Verification items for the finished model (mm, model axes). Face numbers are marked on the shaded views. A direction names the side the tool comes from. Give positions to 0.01 mm unless a question says otherwise; leave off trailing zeros. Loops run counter-clockwise (first coordinate to the right, second up) from the corner with the lowest first, then second, coordinate; pieces in that order, holes last. Notation, with made-up numbers: M 14,0 L 51,0 A31 ccw 51,30 Z; hole C 52,-34.75 d9. An arc over 180 degrees is marked long. Use CSV: the item, a comma, the result in double quotes.
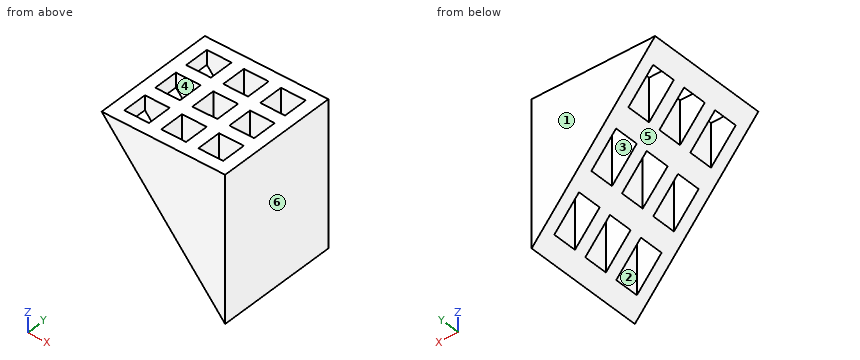
from build123d import *

# Parameters (mm, degrees)
F0_W     = 10
F0_H     = 10
F1_DEPTH = 577
F2_W     = 2
F2_H     = 2
F3_DEPTH = 577.001
F4_W     = 1.9998123646
F4_H     = 2
F4_W_2   = 2
F5_DEPTH = 577.001
F6_DEPTH = 500
F7_DEPTH = 65.276
F9_DEPTH = 10.001


with BuildPart() as f1:
    # F0 (on Top) → F1 (new body)
    with BuildSketch(Plane.XY):
        with Locations((-18.2401322573, 3.4046052024)):
            Rectangle(F0_W, F0_H)
    extrude(amount=F1_DEPTH)

    # F2 (on face) → F3 (cut, through all)
    with BuildSketch(Plane.XY.offset(577)):
        with Locations((-21.2401322573, 6.4046052024)):
            Rectangle(F2_W, F2_H)
        with Locations((-18.2401322573, 6.4046052024)):
            Rectangle(F2_W, F2_H)
        with Locations((-15.2401322573, 6.4046052024)):
            Rectangle(F2_W, F2_H)
        with Locations((-15.2401322573, 0.4046052024)):
            Rectangle(F2_W, F2_H)
        with Locations((-18.2401322573, 0.4046052024)):
            Rectangle(F2_W, F2_H)
        with Locations((-21.2401322573, 0.4046052024)):
            Rectangle(F2_W, F2_H)
    extrude(amount=-F3_DEPTH, mode=Mode.SUBTRACT)

    # F4 (on face) → F5 (cut, through all)
    with BuildSketch(Plane.XY.offset(577)):
        with Locations((-21.2402260751, 3.4046052024)):
            Rectangle(F4_W, F4_H)
        Polygon((-17.2403198928, 4.4376994483), (-19.2403198928, 4.4376994483), (-19.2403198928, 2.4046052024), (-17.2403198928, 2.4376994483), align=None)
        with Locations((-15.2403198928, 3.4074539542)):
            Rectangle(F4_W_2, F4_H)
    extrude(amount=-F5_DEPTH, mode=Mode.SUBTRACT)

    # F6 (cut): a face of the model
    f6_faces = [f1.faces().sort_by_distance(p)[0] for p in [
        (-13.3815536136, 3.4046052024, 577),
    ]]
    extrude(f6_faces, amount=-F6_DEPTH, mode=Mode.SUBTRACT)

    # F7 (cut): a face of the model
    f7_faces = [f1.faces().sort_by_distance(p)[0] for p in [
        (-13.3815536136, 3.4046052024, 77),
    ]]
    extrude(f7_faces, amount=-F7_DEPTH, mode=Mode.SUBTRACT)

    # F8 (on face) → F9 (cut, through all)
    with BuildSketch(Plane(origin=(0, 8.4046052024, 0), x_dir=(-1, 0, 0), z_dir=(0, 1, 0))):
        Polygon((23.2401322573, 0), (23.2401322573, 11.724), (13.2401322573, 0), align=None)
    extrude(amount=-F9_DEPTH, mode=Mode.SUBTRACT)


solid = f1.part
(1) Tool access check on the marked faces 1 and 2. Record the directions out of +Z, -Z, +X, -X, +Y, -Y that give a thin tool (end or side, any length) a straight path to the whole face; none if there is none.
Calculated:
face 1,"+Z, -Z, +X, -X, +Y"
face 2,"+Z, -Z"
(2) Depth check by flat-ended pin: pin 1 Ø5 at (y, z) = (3, 9.5) entering from -X; pin 2 Ø1.5 at (y, z) = (6, 9.5) entering from -X; pin 3 Ø6 at (y, z) = (2, 4.5) entering from -X. Enter the tip coordinate at first touch or a pass-through.
Calculated:
pin 1,"stops at x = -23.24"
pin 2,"stops at x = -21.73"
pin 3,"stops at x = -19.64"
(3) Scan lines: L1, parallel to X at y = 6.5, z = 8.5; L2, parallel to Y at x = -15, z = 2.5; L3, parallel to X at y = 2.75, z = 5.5. Record each from-to range of solid material in increasing order. Write a range as from..to.
Calculated:
L1,"x = -20.24..-19.24, -17.24..-16.24, -14.24..-13.24"
L2,"y = -1.6..-0.6, 1.4..2.41, 4.41..5.4, 7.4..8.4"
L3,"x = -17.24..-16.24, -14.24..-13.24"
(4) Section check A-A on y = 1. Record the cut outline in (x, z), plus the area to 3 significant figures.
Calculated:
outline,"M -23.24,11.72 L -22.24,10.55 L -22.24,11.72 Z; M -20.24,8.21 L -19.24,7.03 L -19.24,11.72 L -20.24,11.72 Z; M -17.24,4.69 L -16.24,3.52 L -16.24,11.72 L -17.24,11.72 Z; M -14.24,1.17 L -13.24,0 L -13.24,11.72 L -14.24,11.72 Z"
area,"23.4 mm²"
(5) Mould release check, pull along X, two halves, no side actions. Record for the marked faces 3, 4, 5 and 6: released by +X, released by -X, zero draft, split by the parting line, or undercut.
Calculated:
face 3,"undercut"
face 4,"undercut"
face 5,"released by -X"
face 6,"released by +X"
(6) Section check B-B on x = -14.75. Record the cut outline in (y, z), plus the area to 3 significant figures.
Calculated:
outline,"M -1.6,1.77 L -0.6,1.77 L -0.6,11.72 L -1.6,11.72 Z; M 1.4,1.77 L 2.41,1.77 L 2.41,11.72 L 1.4,11.72 Z; M 4.41,1.77 L 5.4,1.77 L 5.4,11.72 L 4.41,11.72 Z; M 7.4,1.77 L 8.4,1.77 L 8.4,11.72 L 7.4,11.72 Z"
area,"39.8 mm²"
(7) Section check C-C on z = 5.5. Record the cut outline in (x, y), plus the area to 3 significant figures.
Calculated:
outline,"M -17.93,-1.6 L -13.24,-1.6 L -13.24,8.4 L -17.93,8.4 L -17.93,7.4 L -17.24,7.4 L -17.24,5.4 L -17.93,5.4 L -17.93,4.44 L -17.24,4.44 L -17.24,2.44 L -17.93,2.43 L -17.93,1.4 L -17.24,1.4 L -17.24,-0.6 L -17.93,-0.6 Z; hole M -16.24,-0.6 L -14.24,-0.6 L -14.24,1.4 L -16.24,1.4 Z; hole M -16.24,2.41 L -14.24,2.41 L -14.24,4.41 L -16.24,4.41 Z; hole M -16.24,5.4 L -14.24,5.4 L -14.24,7.4 L -16.24,7.4 Z"
area,"30.8 mm²"
